Check sheet for the modelled part. Datum: model origin and axes. Units: mm. Face numbers are marked on the shaded views. A direction names the side the tool comes from. Coordinates: 2 decimals unless noted, no trailing zeros. Order: outer loops, then holes, each group sorted by start corner. A loop starts at its lowest first (then second) coordinate and runs counter-clockwise, first axis right, second up.
from build123d import *

# Parameters (mm, degrees)
F0_W     = 165.245458
F0_H     = 165.245458
F0_R     = 25.603294
F2_DEPTH = 51.054
F3_R     = 5.08
F1_R     = 76.809882
F1_R_2   = 25.603294
F4_DEPTH = 107.442


with BuildPart() as f2:
    # F0 (on Top) → F2 (new body)
    with BuildSketch(Plane.XY):
        Rectangle(F0_W, F0_H)
        Circle(F0_R, mode=Mode.SUBTRACT)
    extrude(amount=F2_DEPTH)

    # F3
    f3_edges = [f2.edges().sort_by_distance(p)[0] for p in [
        (-82.622729, 0, 51.054),
        (0, -82.622729, 51.054),
        (82.622729, 0, 51.054),
        (0, 82.622729, 51.054),
    ]]
    fillet(f3_edges, radius=F3_R)

    # F1 (on face) → F4 (join)
    with BuildSketch(Plane.XY):
        Circle(F1_R)
        Circle(F1_R_2, mode=Mode.SUBTRACT)
    extrude(amount=F4_DEPTH)


solid = f2.part
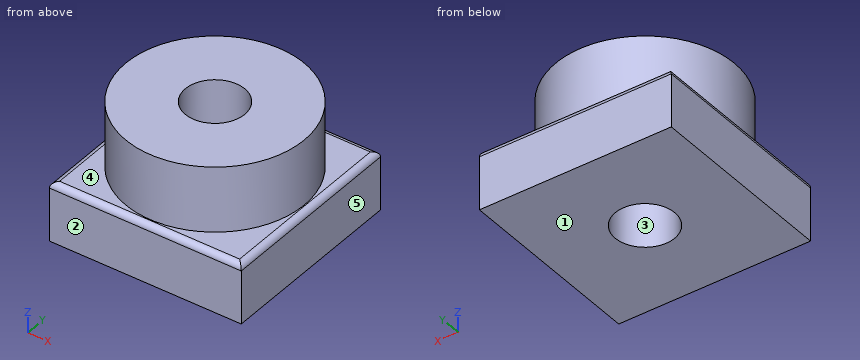
(1) Cross-section at C-C (z = 17.5). Enter the section's corners in (x, y).
Filled in:
outline: (-82.62, -82.62) - (82.62, -82.62) - (82.62, 82.62) - (-82.62, 82.62) - close; hole circle Ø51.21 at (0, 0)
(2) Cross-section at D-D (y = -35.5). Enter the section's corners in (x, z), and give its area (3 significant figures).
Filled in:
outline: (-82.62, 0) - (82.62, 0) - (82.62, 45.97) arc R5.08 ccw to (77.54, 51.05) - (68.11, 51.05) - (68.11, 107.44) - (-68.11, 107.44) - (-68.11, 51.05) - (-77.54, 51.05) arc R5.08 ccw to (-82.62, 45.97) - close
area: 16,100 mm2
(3) Go/stop test with flat-tipped pins: P1, Ø12, axis at x = -25.5, z = 95, coming from the +Y side; P2, Ø3, axis at y = -34.5, z = 96, coming from the +X side; P3, Ø1, axis at x = -41.5, z = 61, coming from the +Y side. Record where each tip stops, or that it passes through.
Filled in:
P1: stops at y = 74.29
P2: stops at x = 69.36
P3: stops at y = 64.95
(4) Release check for a two-part mould opening along Y. For the marked faces 1, 2 and 3 record: +Y half, -Y half, draft (parallel to the pull), parting line (faces both ways), or undercut.
Filled in:
face 1: draft
face 2: -Y half
face 3: undercut
(5) Thickness scan on probe 1 along Y at (x, z) = (0, 65.5); probe 2 along Z at (x, y) = (-64, 70); probe 3 along X at (y, z) = (4.5, 30.5). Record the ranges inside material, lowest first.
Filled in:
probe 1: y = -76.81 to -25.6, 25.6 to 76.81
probe 2: z = 0 to 51.05
probe 3: x = -82.62 to -25.2, 25.2 to 82.62
(6) Cross-section at A-A (x = 0). Enter the section's corners in (y, z), and give its area (3 significant figures).
Filled in:
outline: (-82.62, 0) - (-25.6, 0) - (-25.6, 107.44) - (-76.81, 107.44) - (-76.81, 51.05) - (-77.54, 51.05) arc R5.08 ccw to (-82.62, 45.97) - close; (25.6, 0) - (82.62, 0) - (82.62, 45.97) arc R5.08 ccw to (77.54, 51.05) - (76.81, 51.05) - (76.81, 107.44) - (25.6, 107.44) - close
area: 11,600 mm2
(7) Tool access check on the marked faces 4 and 5. Record the directions out of +Z, -Z, +X, -X, +Y, -Y that give a thin tool (end or side, any length) a straight path to the whole face; none if there is none.
Filled in:
face 4: +Z
face 5: +Z, -Z, +X, +Y, -Y
